```python
from build123d import *

# Parameters (mm, degrees)
FILLET1_R                = 0.01
HEX_2_DEPTH              = 2.08
ESBO_O1_R                = 3
RESSALTO_EXTRUS_O1_DEPTH = 6


with BuildPart() as part:
    # BodySke → BaseBody (revolve)
    with BuildSketch(Plane.XY, mode=Mode.PRIVATE) as basebody_sk:
        with BuildLine():
            Line((20.3, 0), (20.3, 1.6))
            Line((20.3, 1.6), (19.9, 2))
            Line((19.9, 2), (3.3, 2))
            Line((3.3, 2), (3.3, 5.25))
            Line((3.3, 5.25), (2.92, 5.25))
            ThreePointArc((2.92, 5.25), (1.224500646, 4.199464996), (0, 2.625))
            Line((0, 2.625), (0, 0))
            Line((0, 0), (20.3, 0))
        make_face()
    revolve(basebody_sk.sketch.rotate(Axis((0, 0, 0), (1, 0, 0)), 90), axis=Axis((0, 0, 0), (1, 0, 0)))

    # Fillet1
    fillet1_edges = [part.edges().sort_by_distance(p)[0] for p in [
        (3.3, 0, -2),
    ]]
    fillet(fillet1_edges, radius=FILLET1_R)

    # Sketch2 → PreBroach (revolve, cut)
    with BuildSketch(Plane.XY, mode=Mode.PRIVATE) as prebroach_sk:
        Polygon((0, 2), (2.08, 2), (3.234700538, 0), (0, 0), align=None)
    revolve(prebroach_sk.sketch.rotate(Axis((0, 0, 0), (1, 0, 0)), 90), axis=Axis((0, 0, 0), (1, 0, 0)), mode=Mode.SUBTRACT)

    # Sketch3 → Hex 2 (cut)
    with BuildSketch(Plane(origin=(0, 0, 0), x_dir=(0, 0, -1), z_dir=(1, 0, 0))):
        Polygon((-2, -1.154700538), (-2, 1.154700538), (0, 2.309401077), (2, 1.154700538), (2, -1.154700538), (0, -2.309401077), align=None)
    extrude(amount=HEX_2_DEPTH, mode=Mode.SUBTRACT)

    # Esboço1 → Ressalto-extrusão1 (add)
    with BuildSketch(Plane(origin=(3.3, 0, 0), x_dir=(0, 0, -1), z_dir=(1, 0, 0))):
        with Locations(Location((0, 0, 0), (0, 0, 180))):
            Circle(ESBO_O1_R)
    extrude(amount=RESSALTO_EXTRUS_O1_DEPTH)


solid = part.part
```
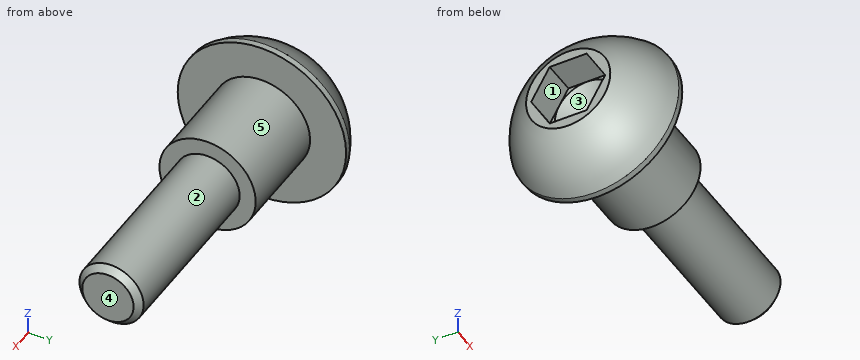
The model under review builds one solid part; all positions refer to its coordinate system, in mm. Face numbers are marked on the shaded views. A direction names the side the tool comes from. Give positions to 0.01 mm unless a question says otherwise; leave off trailing zeros. Write each loop counter-clockwise with the first axis right and the second up, starting at its lowest first coordinate (ties: lowest second). Pieces come first, ordered by that corner, then holes. Notation, with made-up numbers: M 29.5,-13.5 L 36.5,-13.5 A36 ccw 36.5,25.5 Z; hole C -33.75,8 d4. An arc over 180 degrees is marked long. Write item = value, one per line. Start each with the question number.
Q1. Mouldability with a two-part tool opening along Z and no side actions: class the marked faces 3, 4 and 5 as released by +Z, released by -Z, zero draft, split by the parting line, or undercut.
Q2. We need section B-B (x = 18.5). State the section outline as (y, z) points.
Q3. We need section D-D (x = 7.5). State the section outline as (y, z) points, plus the area to 3 significant figures.
Q4. For line 1 (Y direction, x = 13, z = 0); line 2 (Y direction, x = 1.25, z = -0.25); line 3 (Z direction, x = 12.75, y = -1), list the stretches that pass through material, from the lowest coordinate up.
Q5. Clearance check with flat-ended pins moving along their axes: pin 1 (2 mm diameter, centred on y = -4, z = -2, fed in from -X); pin 2 (1 mm diameter, centred on y = 3, z = -1, fed in from -X); pin 3 (0.5 mm diameter, centred on y = 0.5, z = -1.5, fed in from -X). State where each tip first meets the part, or that it passes through.
Q6. We need section A-A (z = -2.25). State the section outline as (x, y) points, plus the area to 3 significant figures.
Q7. Machinability: for the marked faces 1 and 2, which of the approach directions +Z, -Z, +X, -X, +Y, -Y give a long, thin tool a straight path to every point of the face, cutting with its end or side? Answer none if there is none.
Q8. We need section C-C (y = -3.5). State the section outline as (x, z) points, plus the area to 3 significant figures.
Result set:
q1.face_3 = undercut
q1.face_4 = zero draft
q1.face_5 = split by the parting line
q2.outline = C 0,0 d4
q3.outline = C 0,0 d6
q3.area = 28.3 mm2
q4.line_1 = -2 to 2
q4.line_2 = -4.21 to -2.17, 2.17 to 4.21
q4.line_3 = -1.73 to 1.73
q5.pin_1 = 0.55
q5.pin_2 = 0.02
q5.pin_3 = 2.18
q6.outline = M 0,-1.35 A5.18 ccw 2.92,-4.74 L 3.3,-4.74 L 3.3,-1.98 L 9.3,-1.98 L 9.3,1.98 L 3.3,1.98 L 3.3,4.74 L 2.92,4.74 A5.18 ccw 0,1.35 Z
q6.area = 48.3 mm2
q7.face_1 = -X
q7.face_2 = +X
q8.outline = M 2.92,-3.91 L 3.3,-3.91 L 3.3,3.91 L 2.92,3.91 A4.43 ccw Z
q8.area = 16.1 mm2
